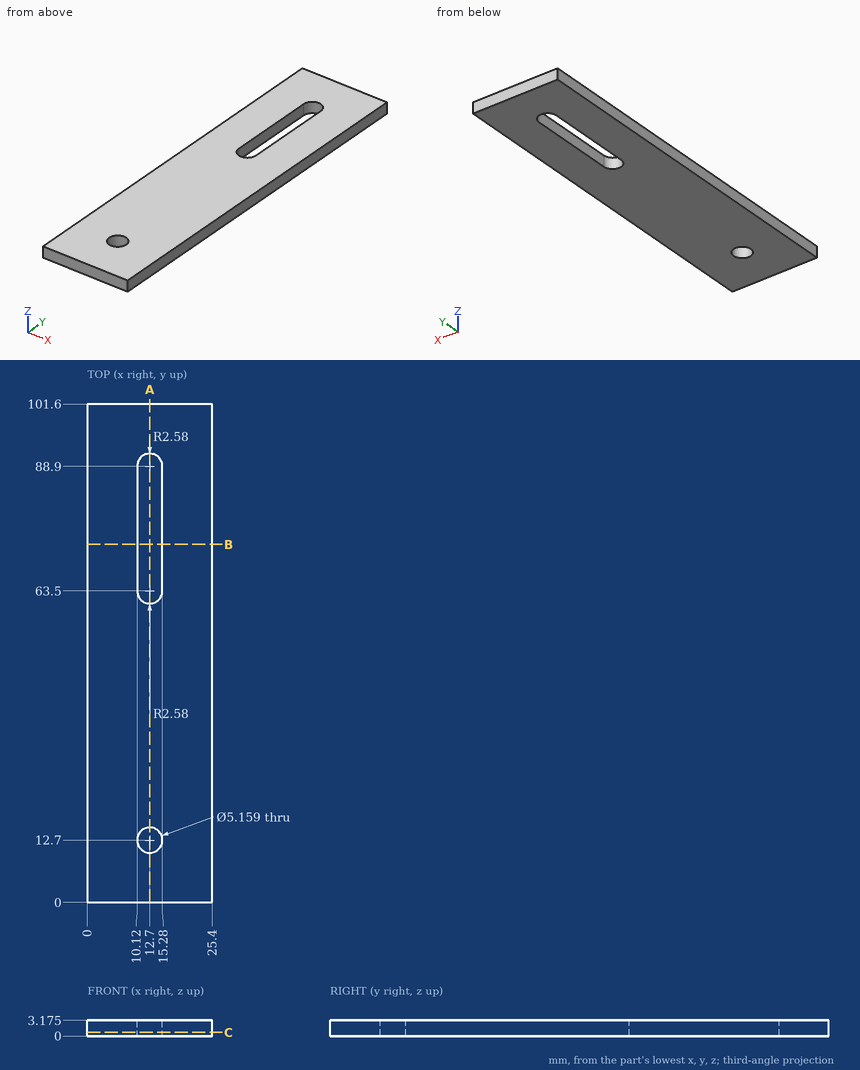
Here's the drawing with two shaded views (mm, measured from the low corner). I have some questions. Coordinates: 2 decimals unless noted, no trailing zeros. Order: outer loops, then holes, each group sorted by start corner. A loop starts at its lowest first (then second) coordinate and runs counter-clockwise, first axis right, second up. Notation, with made-up numbers: (-12, 30) -> (36, 30) arc R20 cw to (36, 53) -> close; hole circle Ø6 at (-29, -5). An arc over 180 degrees is marked (long way). One line per question, with ' | ' between items.
Q1. Imagine slicing it at C-C on z = 0.75. Please give me the cut outline in (x, y).
Return value:
outline: (0, 0) -> (25.4, 0) -> (25.4, 101.6) -> (0, 101.6) -> close; hole circle Ø5.16 at (12.7, 12.7); hole (10.12, 63.5) arc R2.58 ccw to (15.28, 63.5) -> (15.28, 88.9) arc R2.58 ccw to (10.12, 88.9) -> close
Q2. Imagine slicing it at A-A on x = 12.7. Please give me the cut outline in (y, z) (1 decimal).
Return value:
outline: (0, 0) -> (10.1, 0) -> (10.1, 3.2) -> (0, 3.2) -> close; (15.3, 0) -> (60.9, 0) -> (60.9, 3.2) -> (15.3, 3.2) -> close; (91.5, 0) -> (101.6, 0) -> (101.6, 3.2) -> (91.5, 3.2) -> close
Q3. If I drill on L1, parallel to Y at x = 12.7, z = 1.8; L2, parallel to X at y = 69, z = 1.55, over which ranges is the centre line in solid material (lowest first)?
Return value:
L1: 0 to 10.12, 15.28 to 60.92, 91.48 to 101.6 | L2: 0 to 10.12, 15.28 to 25.4
Q4. Imagine slicing it at B-B on y = 73. Please give me the cut outline in (x, z) (1 decimal).
Return value:
outline: (0, 0) -> (10.1, 0) -> (10.1, 3.2) -> (0, 3.2) -> close; (15.3, 0) -> (25.4, 0) -> (25.4, 3.2) -> (15.3, 3.2) -> close
